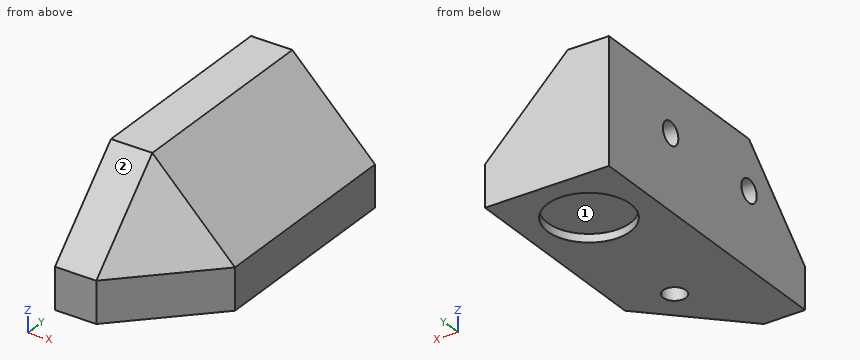
from build123d import *

# Parameters (mm, degrees)
SCHIZZO1_W                   = 30
SCHIZZO1_H                   = 40
ESTRUSIONE_ESTRUSIONE1_DEPTH = 30
SMUSSO1_SIZE                 = 20
ESTRUSIONE_ESTRUSIONE2_DEPTH = 30
FORO_PER_VITE_M5_1_D         = 5.5
FORO_PER_VITE_M5_1_DEPTH     = 15
FORO_PER_VITE_M5_1_TIP       = 1.652366702
FORO_PER_VITE_M5_2_D         = 5.5
FORO_PER_VITE_M5_2_DEPTH     = 15
FORO_PER_VITE_M5_2_TIP       = 1.652366702
SCHIZZO6_R                   = 10
TAGLIO_ESTRUSIONE1_DEPTH     = 2


with BuildPart() as part:
    # Schizzo1 → Estrusione-Estrusione1 (new body)
    with BuildSketch(Plane.XY):
        with Locations((15, 20)):
            Rectangle(SCHIZZO1_W, SCHIZZO1_H)
    extrude(amount=ESTRUSIONE_ESTRUSIONE1_DEPTH)

    # Smusso1
    smusso1_edges = [part.edges().sort_by_distance(p)[0] for p in [
        (30, 20, 30),
        (30, 0, 15),
        (15, 0, 30),
    ]]
    chamfer(smusso1_edges, length=SMUSSO1_SIZE)

    # Schizzo2 → Estrusione-Estrusione2 (add)
    with BuildSketch(Plane(origin=(0, 40, 0), x_dir=(1, 0, 0), z_dir=(0, 1, 0))):
        Polygon((0, 0), (30, 0), (30, -10), (10, -30), (0, -30), align=None)
    extrude(amount=ESTRUSIONE_ESTRUSIONE2_DEPTH)

    # Foro per Vite M5-1
    with Locations(Plane.ZY):
        with Locations((18, 20), (18, 48)):
            Hole(FORO_PER_VITE_M5_1_D / 2, depth=FORO_PER_VITE_M5_1_DEPTH)
            with Locations((0, 0, -(FORO_PER_VITE_M5_1_DEPTH + FORO_PER_VITE_M5_1_TIP / 2))):  # 118° drill point
                Cone(0, FORO_PER_VITE_M5_1_D / 2, FORO_PER_VITE_M5_1_TIP, mode=Mode.SUBTRACT)

    # Foro per Vite M5-2
    with Locations(Plane(origin=(18, 20, 0), x_dir=(-1, 0, 0), z_dir=(0, 0, -1))):
        with Locations((0, 0)):
            Hole(FORO_PER_VITE_M5_2_D / 2, depth=FORO_PER_VITE_M5_2_DEPTH)
            with Locations((0, 0, -(FORO_PER_VITE_M5_2_DEPTH + FORO_PER_VITE_M5_2_TIP / 2))):  # 118° drill point
                Cone(0, FORO_PER_VITE_M5_2_D / 2, FORO_PER_VITE_M5_2_TIP, mode=Mode.SUBTRACT)

    # Schizzo6 → Taglio-Estrusione1 (cut)
    with BuildSketch(Plane(origin=(0, 0, 0), x_dir=(-1, 0, 0), z_dir=(0, 0, -1))):
        with Locations((-15, 55)):
            Circle(SCHIZZO6_R)
    extrude(amount=-TAGLIO_ESTRUSIONE1_DEPTH, mode=Mode.SUBTRACT)


solid = part.part
Read the model definition and answer for the solid it produces. Units are mm, in the model's axes. Face numbers are marked on the shaded views. A direction names the side the tool comes from. Coordinates: 2 decimals unless noted, no trailing zeros. Order: outer loops, then holes, each group sorted by start corner. A loop starts at its lowest first (then second) coordinate and runs counter-clockwise, first axis right, second up. Notation, with made-up numbers: M 43.5,86.25 L 91.5,86.25 A28 ccw 91.5,117.25 Z; hole C 54,63 d1. An arc over 180 degrees is marked long. Put each result on its own line as item: value. Start each with the question number.
Item 1: Section C-C, the plane x = 13 is taken. Determine the outline of the cut face in (y, z), plus the area to 3 significant figures.
Item 2: For the marked faces 1 and 2, determine the directions among +Z, -Z, +X, -X, +Y, -Y from which every point of the face is accessible in a straight line to the end or side of a thin tool.
Item 3: Given pin 1 Ø7 at (y, z) = (48, 18) entering from +X; pin 2 Ø1.5 at (x, z) = (25, 7) entering from -Y; pin 3 Ø10 at (x, y) = (13, 52) entering from -Z, each flat-ended and moving along its own axis, determine where each tip first touches the part or whether it passes through.
Item 4: Section D-D, the plane x = 22 is taken. Determine the outline of the cut face in (y, z).
Item 5: Consider probe 1 along Z at (x, y) = (7.75, 20); probe 2 along Y at (x, z) = (11.5, 20); probe 3 along Y at (x, z) = (7.75, 18). Determine where each line is inside the solid, lowest interval first. Write a range as [from, to].
Item 6: Section B-B, the plane z = 13 is taken. Determine the outline of the cut face in (x, y).
Item 7: Section A-A, the plane y = 55 is taken. Determine the outline of the cut face in (x, z).
Computed:
1. outline: M 3,0 L 45.2,0 L 45.2,2 L 64.8,2 L 64.8,0 L 70,0 L 70,27 L 20,27 L 3,10 Z; hole C 20,18 d5.5; hole C 48,18 d5.5
1. area: 1,580 mm2
2. face 1: -Z
2. face 2: +Z, +X, -X, -Y
3. pin 1: stops at x = 25.5
3. pin 2: stops at y = 14.25
3. pin 3: stops at z = 2
4. outline: M 12,0 L 47.86,0 L 47.86,2 L 62.14,2 L 62.14,0 L 70,0 L 70,18 L 20,18 L 12,10 Z
5. probe 1: z = [0, 15.25], [20.75, 30]
5. probe 2: y = [11.5, 18.11], [21.89, 46.11], [49.89, 70]
5. probe 3: y = [8, 17.25], [22.75, 45.25], [50.75, 70]
6. outline: M 0,3 L 10,3 L 27,20 L 27,70 L 0,70 Z; hole C 18,20 d5.5
7. outline: M 0,0 L 5,0 L 5,2 L 25,2 L 25,0 L 30,0 L 30,10 L 10,30 L 0,30 Z
